The listing builds one solid part. Answer for the finished solid, in the listing's coordinates (mm). Give positions to 0.01 mm unless a question says otherwise; leave off trailing zeros. Write each loop counter-clockwise with the first axis right and the second up, starting at its lowest first coordinate (ties: lowest second). Pieces come first, ordered by that corner, then holes. Notation, with made-up numbers: (-23.5, 74) - (15.5, 74) arc R9 ccw to (15.5, 79) - close; hole circle Ø9 at (-21.5, 58.5). An arc over 180 degrees is marked (long way). Use a Markdown table: item, result. Add a question column.
from build123d import *

# Parameters (mm, degrees)
SKETCH1_R           = 5
BOSS_EXTRUDE1_DEPTH = 2.5


with BuildPart() as part:
    # Sketch1 → Boss-Extrude1 (new, symmetric)
    with BuildSketch(Plane.XY):
        with BuildLine():
            Line((0, 25), (140, 25))
            Line((140, 25), (203.998392257, -4.842940419))
            Line((203.998392257, -4.842940419), (205.789355906, -15))
            Line((205.789355906, -15), (202.289355906, -19))
            Line((202.289355906, -19), (198.789355906, -15))
            Line((198.789355906, -15), (195.289355906, -19))
            Line((195.289355906, -19), (191.789355906, -15))
            Line((191.789355906, -15), (188.289355906, -19))
            Line((188.289355906, -19), (184.789355906, -15))
            Line((184.789355906, -15), (181.289355906, -19))
            Line((181.289355906, -19), (177.789355906, -15))
            Line((177.789355906, -15), (174.289355906, -19))
            Line((174.289355906, -19), (170.789355906, -15))
            ThreePointArc((170.789355906, -15), (138.414706816, 12.155175392), (111, -20))
            Line((111, -20), (90, -20))
            ThreePointArc((90, -20), (84.142135624, -5.857864376), (70, 0))
            Line((70, 0), (0, 0))
            ThreePointArc((0, 0), (-12.5, 12.5), (0, 25))
        make_face()
        with Locations((75, 12.5)):
            Circle(SKETCH1_R, mode=Mode.SUBTRACT)
        with Locations((0, 12.5)):
            Circle(SKETCH1_R, mode=Mode.SUBTRACT)
    extrude(amount=BOSS_EXTRUDE1_DEPTH, both=True)


solid = part.part
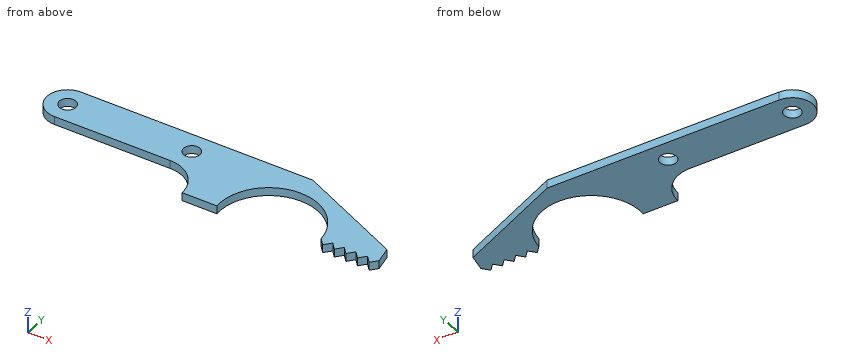
1. The part is cut by section C-C (x = 75). Give the vertices of the cut face in (y, z).
2. Given P1, Ø6, axis at x = 0, y = 12.5, coming from the -Z side; P2, Ø2.5, axis at x = 37, z = -0.5, coming from the -Y side, each flat-ended and moving along its own axis, determine where each tip first touches the part or whether it passes through.
3. The part is cut by section D-D (x = 168). Give the vertices of the cut face in (y, z).
4. The part is cut by section A-A (z = -1.1). Give the vertices of the cut face in (x, y), and give its area (3 significant figures).
5. Consider L1, parallel to Y at x = 0, z = 0.8; L2, parallel to X at y = 10, z = -1.25; L3, parallel to X at y = 15, z = -1.3. Determine where each line is inside the solid, lowest interval first. Write a range as [from, to].
6. The part is cut by section B-B (y = 4.5). Give the vertices of the cut face in (x, z), and give its area (4 significant figures).
Check values:
| question | item | result |
|---|---|---|
| 1 | outline | (-0.64, -2.5) - (7.5, -2.5) - (7.5, 2.5) - (-0.64, 2.5) - close; (17.5, -2.5) - (25, -2.5) - (25, 2.5) - (17.5, 2.5) - close |
| 2 | P1 | passes through |
| 2 | P2 | stops at y = 0 |
| 3 | outline | (-4.84, -2.5) - (11.94, -2.5) - (11.94, 2.5) - (-4.84, 2.5) - close |
| 4 | outline | (0, 0) - (70, 0) arc R20 cw to (90, -20) - (111, -20) arc R30 cw to (170.79, -15) - (174.29, -19) - (177.79, -15) - (181.29, -19) - (184.79, -15) - (188.29, -19) - (191.79, -15) - (195.29, -19) - (198.79, -15) - (202.29, -19) - (205.79, -15) - (204, -4.84) - (140, 25) - (0, 25) arc R12.5 ccw to start; hole circle Ø10 at (0, 12.5); hole circle Ø10 at (75, 12.5) |
| 4 | area | 4,960 mm2 |
| 5 | L1 | y = [0, 7.5], [17.5, 25] |
| 5 | L2 | x = [-12.25, -4.33], [4.33, 70.67], [79.33, 129.49], [152.34, 172.17] |
| 5 | L3 | x = [-12.25, -4.33], [4.33, 70.67], [79.33, 161.45] |
| 6 | outline | (-9.6, -2.5) - (120.78, -2.5) - (120.78, 2.5) - (-9.6, 2.5) - close; (161.05, -2.5) - (183.96, -2.5) - (183.96, 2.5) - (161.05, 2.5) - close |
| 6 | area | 766.5 mm2 |
